Part model, mm, in its own coordinate system. Face numbers are marked on the shaded views. A direction names the side the tool comes from. Give positions to 0.01 mm unless a question says otherwise; leave off trailing zeros. Write each loop counter-clockwise with the first axis right and the second up, starting at its lowest first coordinate (ties: lowest second). Pieces come first, ordered by that corner, then holes. Notation, with made-up numbers: M 62,2.5 L 70,2.5 A9 ccw 70,8.5 Z; hole C 65.25,47.25 d8. An arc over 180 degrees is marked long. Use a Markdown table: item, result. Add a question column.
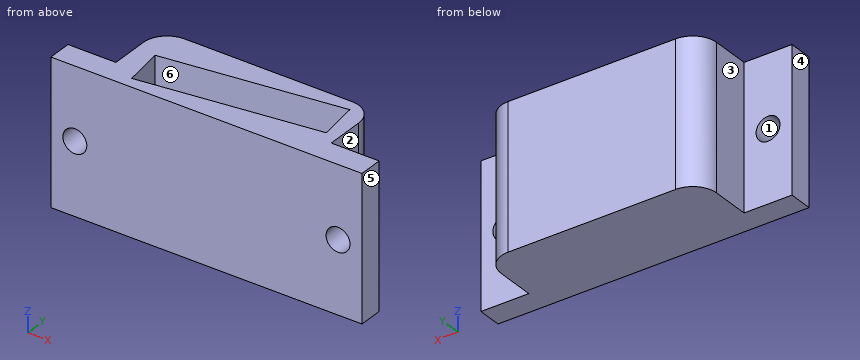
from build123d import *

# Parameters (mm, degrees)
F1_DEPTH = 30
F2_DEPTH = 3
F3_R     = 5
F5_R     = 2.5
F4_R     = 2.5
F6_DEPTH = 25


with BuildPart() as f1:
    # F0 (on Top) → F1 (new body)
    with BuildSketch(Plane.XY):
        Polygon((-32.5, -9), (32.5, -9), (32.5, -4), (22.5, -4), (22.5, 9), (-22.5, 9), (-22.5, -4), (-32.5, -4), align=None)
        Polygon((18.7564, 6.652187), (19.862741, -1.775506), (-17.318257, -6.656426), (-18.424599, 1.771267), align=None, mode=Mode.SUBTRACT)
    extrude(amount=F1_DEPTH)

    # F0 (on Top) → F2 (join)
    with BuildSketch(Plane.XY):
        Polygon((-17.318257, -6.656426), (19.862741, -1.775506), (18.7564, 6.652187), (-18.424599, 1.771267), align=None)
    extrude(amount=F2_DEPTH)

    # F3
    f3_edges = [f1.edges().sort_by_distance(p)[0] for p in [
        (22.5, 9, 15),
        (-22.5, 9, 15),
    ]]
    fillet(f3_edges, radius=F3_R)

    # F5 (on face) + F4 (on face) → F6 (cut)
    with BuildSketch(Plane(origin=(0, -4, 0), x_dir=(-1, 0, 0), z_dir=(0, 1, 0))):
        with Locations((27.5, 15)):
            Circle(F5_R)
    with BuildSketch(Plane(origin=(0, -4, 0), x_dir=(-1, 0, 0), z_dir=(0, 1, 0))):
        with Locations((-27.5, 15)):
            Circle(F4_R)
    extrude(amount=-F6_DEPTH, mode=Mode.SUBTRACT)


solid = f1.part
1. Cut at C-C (z = 11.25). Write the cut outline in (x, y).
2. Mould opens along X. For the marked faces 4, 5 and 6 say: released by +X, released by -X, zero draft, split by the parting line, or undercut.
3. Cut at B-B (x = -27.5). Write the cut outline in (y, z), then the cut area to 3 significant figures.
4. Tool access for the marked faces 1, 2 and 3: list every direction of +Z, -Z, +X, -X, +Y, -Y with a clear straight run to the whole face (end or side of a thin tool).
5. Flat gauge pins, fed straight in: pin 1 (2 mm diameter, centred on y = 2, z = 5, fed in from +X); pin 2 (3 mm diameter, centred on y = 5, z = 6.5, fed in from -X); pin 3 (3 mm diameter, centred on x = -27, z = 16.5, fed in from +Y). Where does each tip first touch, or does it go through?
6. Cut at A-A (z = 15). Write the cut outline in (x, y).
7. Drill centre lines: probe 1 along Z at (x, y) = (-27.5, -6.7); probe 2 along Y at (x, z) = (-24, 11.5); probe 3 along X at (y, z) = (0, 9.75). Where is each one in solid material? Low to high. Write a range as [from, to].
8. Cut at D-D (x = -6.5). Write the cut outline in (y, z).
A:
| question | item | result |
|---|---|---|
| 1 | outline | M -32.5,-9 L 32.5,-9 L 32.5,-4 L 22.5,-4 L 22.5,4 A5 ccw 17.5,9 L -17.5,9 A5 ccw -22.5,4 L -22.5,-4 L -32.5,-4 Z; hole M -18.42,1.77 L -17.32,-6.66 L 19.86,-1.78 L 18.76,6.65 Z |
| 2 | face 4 | released by -X |
| 2 | face 5 | released by +X |
| 2 | face 6 | undercut |
| 3 | outline | M -9,0 L -4,0 L -4,12.5 L -9,12.5 Z; M -9,17.5 L -4,17.5 L -4,30 L -9,30 Z |
| 3 | area | 125 mm² |
| 4 | face 1 | +Y, -Y |
| 4 | face 2 | +Z, -Z, +X, +Y |
| 4 | face 3 | +Z, -Z, -X, +Y |
| 5 | pin 1 | stops at x = 22.5 |
| 5 | pin 2 | stops at x = -22.5 |
| 5 | pin 3 | stops at y = -4 |
| 6 | outline | M -32.5,-9 L -30,-9 L -30,-4 L -32.5,-4 Z; M -25,-9 L 25,-9 L 25,-4 L 22.5,-4 L 22.5,4 A5 ccw 17.5,9 L -17.5,9 A5 ccw -22.5,4 L -22.5,-4 L -25,-4 Z; M 30,-9 L 32.5,-9 L 32.5,-4 L 30,-4 Z; hole M -18.42,1.77 L -17.32,-6.66 L 19.86,-1.78 L 18.76,6.65 Z |
| 7 | probe 1 | z = [0, 12.5], [17.5, 30] |
| 7 | probe 2 | y = [-9, -4] |
| 7 | probe 3 | x = [-22.5, -18.19], [19.63, 22.5] |
| 8 | outline | M -9,0 L 9,0 L 9,30 L 3.34,30 L 3.34,3 L -5.24,3 L -5.24,30 L -9,30 Z |
